```python
from build123d import *

# Parameters (mm, degrees)
SKETCH1_R                                            = 50
BOSS_EXTRUDE1_DEPTH                                  = 10
CBORE_FOR_M6_HEX_SOCKET_HEAD_CAP_SCREW1_D            = 5.5
CBORE_FOR_M6_HEX_SOCKET_HEAD_CAP_SCREW1_CBORE_D      = 12
CBORE_FOR_M6_HEX_SOCKET_HEAD_CAP_SCREW1_CBORE_DEPTH  = 3
F_12_0_12_DIAMETER_HOLE1_D                           = 12
CSK_FOR_M3_HEX_SOCKET_COUNTERSUNK_CAP_SC_D           = 5.5
CSK_FOR_M3_HEX_SOCKET_COUNTERSUNK_CAP_SC_CSINK_D     = 11.2
CSK_FOR_M3_HEX_SOCKET_COUNTERSUNK_CAP_SC_CSINK_ANGLE = 90
CHAMFER1_SIZE                                        = 1


with BuildPart() as part:
    # Sketch1 → Boss-Extrude1 (new body)
    with BuildSketch(Plane.XY):
        Circle(SKETCH1_R)
    extrude(amount=BOSS_EXTRUDE1_DEPTH)

    # CBORE for M6 Hex Socket Head Cap Screw1 (through all)
    with Locations(Plane.XY.offset(10)):
        with Locations((-32.5, 21), (32.5, 21), (32.5, -21), (-32.5, -21)):
            CounterBoreHole(CBORE_FOR_M6_HEX_SOCKET_HEAD_CAP_SCREW1_D / 2, CBORE_FOR_M6_HEX_SOCKET_HEAD_CAP_SCREW1_CBORE_D / 2, CBORE_FOR_M6_HEX_SOCKET_HEAD_CAP_SCREW1_CBORE_DEPTH)

    # Ø12.0 (12) Diameter Hole1 (through all)
    with Locations(Plane.XY.offset(10)):
        with Locations((0, 33.07), (0, -33.07)):
            Hole(F_12_0_12_DIAMETER_HOLE1_D / 2)

    # CSK for M3 Hex Socket Countersunk Cap Screw1 (through all)
    with Locations(Plane(origin=(0, 0, 0), x_dir=(-1, 0, 0), z_dir=(0, 0, -1))):
        with Locations((-32.5, 21), (-32.5, -21), (32.5, -21), (32.5, 21)):
            CounterSinkHole(CSK_FOR_M3_HEX_SOCKET_COUNTERSUNK_CAP_SC_D / 2, CSK_FOR_M3_HEX_SOCKET_COUNTERSUNK_CAP_SC_CSINK_D / 2, counter_sink_angle=CSK_FOR_M3_HEX_SOCKET_COUNTERSUNK_CAP_SC_CSINK_ANGLE)

    # Chamfer1
    chamfer1_edges = [part.edges().sort_by_distance(p)[0] for p in [
        (-50, 0, 0),
        (-50, 0, 10),
    ]]
    chamfer(chamfer1_edges, length=CHAMFER1_SIZE)


solid = part.part
```
Geometry check sheet. Reference: the model listing, model coordinates, mm. A direction names the side the tool comes from. Give positions to 0.01 mm unless a question says otherwise; leave off trailing zeros. Write each loop counter-clockwise with the first axis right and the second up, starting at its lowest first coordinate (ties: lowest second). Pieces come first, ordered by that corner, then holes.
1) Section check A-A, the plane z = 5.5. Record the boundary of the cut face in (x, y).
2) Gauge pin test, flat ends, axial feed: pin 1 (11 mm diameter, centred on x = -32.5, y = -21, fed in from +Z); pin 2 (13 mm diameter, centred on x = 29.5, y = -23, fed in from +Z); pin 3 (9 mm diameter, centred on x = -32.5, y = -21, fed in from -Z); pin 4 (7 mm diameter, centred on x = 32.5, y = -21, fed in from -Z). Record the tip position at first contact, or that the pin passes through.
3) Section check C-C, the plane y = 21. State how many separate pieces and enclosed holes the cut face has, and give its area (3 significant figures).
4) Section check B-B, the plane x = 0. Record the boundary of the cut face in (y, z).
5) Material ranges on L1, parallel to Y at x = 32.5, z = 9.25; L2, parallel to Y at x = 32.5, z = 8.6; L3, parallel to X at y = 17.5, z = 8.75, recorded low to high.
6) Access from +Z, -Z, +X, -X, +Y, -Y to the whole of each face (thin tool, end or side, straight path). Record for faces 1 (the conical face through (35.255, 21.868, 2.712)), 2 (the flat face through (34, -24, 7)).
Computed:
1. outline: circle Ø100 at (0, 0); hole circle Ø5.5 at (-32.5, -21); hole circle Ø5.5 at (-32.5, 21); hole circle Ø12 at (0, -33.07); hole circle Ø12 at (0, 33.07); hole circle Ø5.5 at (32.5, -21); hole circle Ø5.5 at (32.5, 21)
2. pin 1: stops at z = 7
2. pin 2: stops at z = 10
2. pin 3: stops at z = 1.1
2. pin 4: stops at z = 2.1
3. separate pieces: 3
3. enclosed holes: 0
3. area: 740 mm2
4. outline: (-50, 1) - (-49, 0) - (-39.07, 0) - (-39.07, 10) - (-49, 10) - (-50, 9) - close; (-27.07, 0) - (27.07, 0) - (27.07, 10) - (-27.07, 10) - close; (39.07, 0) - (49, 0) - (50, 1) - (50, 9) - (49, 10) - (39.07, 10) - close
5. L1: y = -37.67 to -27, -15 to 15, 27 to 37.67
5. L2: y = -38 to -27, -15 to 15, 27 to 38
5. L3: x = -46.84 to -37.37, -27.63 to 27.63, 37.37 to 46.84
6. face 1: -Z
6. face 2: +Z
